Could you check a few things on this model? Use its own coordinates, in mm. Face numbers are marked on the shaded views. A direction names the side the tool comes from. Round coordinates to 2 decimals unless told otherwise and drop trailing zeros. Order: outer loops, then holes, each group sorted by start corner. A loop starts at its lowest first (then second) coordinate and runs counter-clockwise, first axis right, second up. Notation, with made-up numbers: (11, -8) -> (61, -8) arc R33 cw to (61, 22) -> close; hole circle Ø11 at (59.25, 77). An arc over 180 degrees is marked (long way). One line per question, with ' | ' between items.
```python
from build123d import *

# Parameters (mm, degrees)
SKETCH_1_R      = 1.6
EXTRUDE_1_DEPTH = 2
SKETCH_3_W      = 6
SKETCH_3_H      = 6
EXTRUDE_3_DEPTH = 130
SKETCH_4_W      = 3.5
SKETCH_4_H      = 6
EXTRUDE_4_DEPTH = 3
EXTRUDE_6_DEPTH = 2


with BuildPart() as part:
    # 草图1 → 凸台-拉伸1 (new body)
    with BuildSketch(Plane(origin=(0, 0, 0), x_dir=(1, 0, 0), z_dir=(0, 1, 0))):
        with BuildLine():
            ThreePointArc((8.06014642, -3.856953405), (11, 0), (8.06014642, 3.856953405))
            ThreePointArc((8.06014642, 3.856953405), (3.36087852, 5.821212354), (-0.68985358, 8.90876826))
            ThreePointArc((-0.68985358, 8.90876826), (-5.5, 9.526279442), (-7.37029284, 5.051814855))
            ThreePointArc((-7.37029284, 5.051814855), (-6.721757039, 0), (-7.37029284, -5.051814855))
            ThreePointArc((-7.37029284, -5.051814855), (-5.5, -9.526279442), (-0.68985358, -8.90876826))
            ThreePointArc((-0.68985358, -8.90876826), (3.36087852, -5.821212354), (8.06014642, -3.856953405))
        make_face()
        with Locations(Location((7, 0, 0), (0, 0, 270))):
            Circle(SKETCH_1_R, mode=Mode.SUBTRACT)
        with Locations(Location((-3.5, -6.062177826, 0), (0, 0, 270))):
            Circle(SKETCH_1_R, mode=Mode.SUBTRACT)
        with Locations(Location((-3.5, 6.062177826, 0), (0, 0, 270))):
            Circle(SKETCH_1_R, mode=Mode.SUBTRACT)
    extrude(amount=EXTRUDE_1_DEPTH)

    # 草图3 → 凸台-拉伸3 (add)
    with BuildSketch(Plane(origin=(0, 0, 0), x_dir=(1, 0, 0), z_dir=(0, 1, 0))):
        with Locations((-4.5, 0)):
            Rectangle(SKETCH_3_W, SKETCH_3_H)
    extrude(amount=EXTRUDE_3_DEPTH)

    # 草图4 → 凸台-拉伸4 (add)
    with BuildSketch(Plane(origin=(0, 130, 0), x_dir=(1, 0, 0), z_dir=(0, 1, 0))):
        with Locations((-5.75, 0)):
            Rectangle(SKETCH_4_W, SKETCH_4_H)
    extrude(amount=EXTRUDE_4_DEPTH)

    # 草图5 → 凸台-拉伸6 (add)
    with BuildSketch(Plane(origin=(0, 2, 0), x_dir=(1, 0, 0), z_dir=(0, 1, 0))):
        Polygon((-7.5, 6.062177826), (-7.5, -6.062177826), (-7.5, -10.062177826), (-3.5, -10.062177826), (-6.276889943, -8.064926479), (-6.276889943, 5.727222141), (-3.5, 10.062177826), (-7.5, 10.062177826), align=None)
    extrude(amount=-EXTRUDE_6_DEPTH)


solid = part.part
```
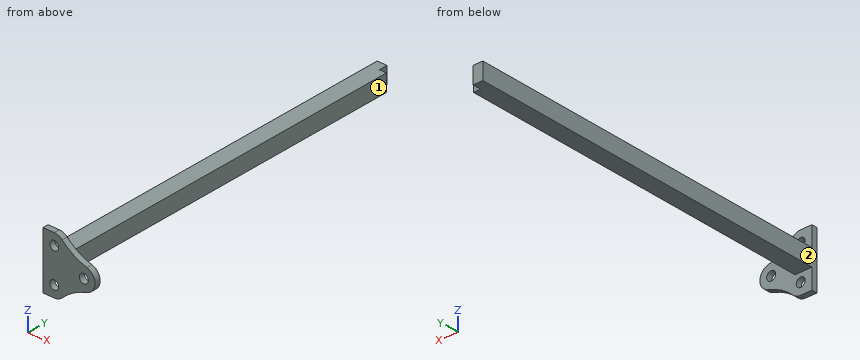
1. I want a section at B-B on y = 111. List the corners of the cut face in (x, z) for me.
From the geometry:
outline: (-7.5, -3) -> (-1.5, -3) -> (-1.5, 3) -> (-7.5, 3) -> close
2. I'm going to push flat-ended pins straight in: pin 1 (2.5 mm diameter, centred on y = 132, z = -0.5, fed in from +X); pin 2 (9 mm diameter, centred on x = 6, z = -4.5, fed in from +Y); pin 3 (4 mm diameter, centred on x = -3.5, z = -6.06, fed in from -Y); pin 4 (1.9 mm diameter, centred on x = -3.5, z = 6.06, fed in from +Y). Where does each tip first touch, or does it pass through?
From the geometry:
pin 1: stops at x = -4 | pin 2: stops at y = 2 | pin 3: stops at y = 0 | pin 4: passes through
3. I want a section at A-A on z = 0. List the corners of the cut face in (x, y) for me.
From the geometry:
outline: (-7.5, 0) -> (5.4, 0) -> (5.4, 2) -> (-1.5, 2) -> (-1.5, 130) -> (-4, 130) -> (-4, 133) -> (-7.5, 133) -> close; (8.6, 0) -> (11, 0) -> (11, 2) -> (8.6, 2) -> close
4. On a 3-axis mill with a long thin cutter (end or side, diameter ignored), from which of +Z, -Z, +X, -X, +Y, -Y can I reach the whole of each face in a straight line? I mean the marked faces 1 and 2. Say none if no direction works.
From the geometry:
face 1: +Z, -Z, +X, +Y | face 2: +Z, -Z, -X, +Y, -Y
5. I want a section at C-C on x = 1.5. List the corners of the cut face in (y, z) for me, and give its area (3 significant figures).
From the geometry:
outline: (0, -7.04) -> (2, -7.04) -> (2, 7.04) -> (0, 7.04) -> close | area: 28.2 mm²
6. I need wall thicknesses on probe 1 along X at (y, z) = (1.1, 0); probe 2 along Z at (x, y) = (-3.5, 113.5); probe 3 along Y at (x, z) = (-3.75, 2.5). Which ranges of each line are inside material? Lowest first, please.
From the geometry:
probe 1: x = -7.5 to 5.4, 8.6 to 11 | probe 2: z = -3 to 3 | probe 3: y = 0 to 130
